Read the model definition and answer for the solid it produces. Units are mm, in the model's axes. A direction names the side the tool comes from. Give positions to 0.01 mm unless a question says otherwise; leave off trailing zeros. Order: outer loops, then holes, each group sorted by start corner. A loop starts at its lowest first (then second) coordinate and runs counter-clockwise, first axis right, second up. Notation, with made-up numbers: M 54.5,24 L 84.5,24 A34 ccw 84.5,62 Z; hole C 47.25,62.5 d3. An arc over 180 degrees is marked long. Write item = value, one per line. Start each with the question number.
from build123d import *

# Parameters (mm, degrees)
SKETCH_1_R          = 40
EXTRUDE_1_DEPTH     = 12
SKETCH_2_R          = 5
SKETCH_2_R_2        = 2.5
CUT_EXTRUDE_1_DEPTH = 10
SKETCH_3_R          = 4.75
CUT_EXTRUDE_2_DEPTH = 5


with BuildPart() as part:
    # 草图1 → 凸台-拉伸1 (new body)
    with BuildSketch(Plane.XY):
        Circle(SKETCH_1_R)
    extrude(amount=EXTRUDE_1_DEPTH)

    # 草图2 → 切除-拉伸1 (cut)
    with BuildSketch(Plane.XY.offset(12)):
        Circle(SKETCH_2_R)
        with Locations((0, 30)):
            Circle(SKETCH_2_R_2)
        with Locations((0, -30)):
            Circle(SKETCH_2_R_2)
    extrude(amount=-CUT_EXTRUDE_1_DEPTH, mode=Mode.SUBTRACT)

    # 草图3 → 切除-拉伸2 (cut)
    with BuildSketch(Plane(origin=(0, 0, 0), x_dir=(-1, 0, 0), z_dir=(0, 0, -1))):
        with Locations((0, -30)):
            Circle(SKETCH_3_R)
        with Locations((0, 30)):
            Circle(SKETCH_3_R)
    extrude(amount=-CUT_EXTRUDE_2_DEPTH, mode=Mode.SUBTRACT)


solid = part.part
1) Each of these flat-tipped pins is pushed along its axis until it touches: P1, Ø4, axis at y = 20, z = 9, coming from the -X side; P2, Ø5, axis at x = -11.5, z = 10, coming from the +Y side; P3, Ø4, axis at x = 0, y = -30, coming from the +Z side; P4, Ø3, axis at x = -16, z = 1.5, coming from the +Y side. Where does it stop, or does it pass through?
2) For a pull along X with two mould halves and no side action, classify faces 4 (the face through (-2, -32, 5)), 5 (the face through (-8.67, -39.05, 5.92)), 6 (the face through (1.34, 32.11, 8.55)), 7 (the face through (-1, 1, 0)) as pulls with the +X half, pulls with the -X half, needs draft (parallel to the pull), parting line crosses it, or undercut.
3) Find section D-D on y = 0. Determine the outline of the cut face in (x, z), plus the area to 3 significant figures.
4) Find section B-B on z = 11. Determine the outline of the cut face in (x, y), plus the area to 3 significant figures.
5) Find section C-C on y = -30. Determine the outline of the cut face in (x, z).
6) Find the intervals of material crossed by probe 1 along Y at (x, z) = (0, 2.75); probe 2 along Y at (x, z) = (0, 8); probe 3 along Y at (x, z) = (3, 6.75), in increasing order. Write a range as [from, to].
7) Find section A-A on x = 0. Determine the outline of the cut face in (y, z).
8) For faces 1 (the face through (1.03, -34.637, 2.465)), 2 (the face through (8, 1, 12)), 3 (the face through (0, 0, 2)), determine the directions among +Z, -Z, +X, -X, +Y, -Y from which every point of the face is accessible in a straight line to the end or side of a thin tool.
Numbers:
q1.P1 = -35.72
q1.P2 = 38.97
q1.P3 = through
q1.P4 = 37.28
q2.face_4 = undercut
q2.face_5 = parting line crosses it
q2.face_6 = undercut
q2.face_7 = needs draft
q3.outline = M -40,0 L 40,0 L 40,12 L 5,12 L 5,2 L -5,2 L -5,12 L -40,12 Z
q3.area = 860 mm2
q4.outline = C 0,0 d80; hole C 0,0 d10; hole C 0,-30 d5; hole C 0,30 d5
q4.area = 4,910 mm2
q5.outline = M -26.46,0 L -4.75,0 L -4.75,5 L -2.5,5 L -2.5,12 L -26.46,12 Z; M 2.5,5 L 4.75,5 L 4.75,0 L 26.46,0 L 26.46,12 L 2.5,12 Z
q6.probe_1 = [-40, -34.75], [-25.25, -5], [5, 25.25], [34.75, 40]
q6.probe_2 = [-40, -32.5], [-27.5, -5], [5, 27.5], [32.5, 40]
q6.probe_3 = [-39.89, -4], [4, 39.89]
q7.outline = M -40,0 L -34.75,0 L -34.75,5 L -32.5,5 L -32.5,12 L -40,12 Z; M -27.5,5 L -25.25,5 L -25.25,0 L 25.25,0 L 25.25,5 L 27.5,5 L 27.5,12 L 5,12 L 5,2 L -5,2 L -5,12 L -27.5,12 Z; M 32.5,5 L 34.75,5 L 34.75,0 L 40,0 L 40,12 L 32.5,12 Z
q8.face_1 = -Z
q8.face_2 = +Z, +X, -X, +Y, -Y
q8.face_3 = +Z
